Build history of the part. All positions in model axes, mm. Give positions to 0.01 mm unless a question says otherwise; leave off trailing zeros. Loops run counter-clockwise (first coordinate to the right, second up) from the corner with the lowest first, then second, coordinate; pieces in that order, holes last. Notation, with made-up numbers: M 38.5,-34 L 73.5,-34 A38 ccw 73.5,4 Z; hole C -34,-22 d1. An arc over 180 degrees is marked long. Answer as a JSON object with one key per item and string values. Group by question number.
1. Drop flat-ended pins along their axis: pin 1 Ø1.5 at (x, y) = (85, 3.5) entering from -Z; pin 2 Ø1.5 at (x, y) = (11.5, 3.5) entering from -Z; pin 3 Ø1.5 at (y, z) = (1, 7) entering from -X. Give the stop position or say it passes through.
2. Slice it at A-A (y = 3.1). Give the number of separate pieces and of enclosed holes in the cut face, then the cut area to 3 significant figures.
3. Drill centre lines: line 1 along X through (y, z) = (2.25, 0); line 2 along X through (y, z) = (0.9, 7); line 3 along X through (y, z) = (3.75, -6). Where is each one in solid material? Low to high. Write a range as [from, to].
4. Slice it at B-B (x = -36.5). List the corners of the cut face in (y, z), then the cut area to 3 significant figures.
from build123d import *

# Parameters (mm, degrees)
BOSS_EXTRUDE1_DEPTH = 5
SKETCH2_R           = 4
SKETCH2_R_2         = 1.5
CUT_EXTRUDE1_DEPTH  = 5
SKETCH3_R           = 1.5
CUT_EXTRUDE2_DEPTH  = 5
FILLET3_R           = 10
FILLET4_R           = 10


with BuildPart() as part:
    # Sketch1 → Boss-Extrude1 (new body)
    with BuildSketch(Plane(origin=(0, 0, 0), x_dir=(1, 0, 0), z_dir=(0, 1, 0))):
        Polygon((-85.638593384, 10), (-100, 10), (-100, -10), (-85.638593384, -10), (70, -10), (70, -15), (100, -15), (100, -10), (100, 10), (100, 15), (70, 15), (70, 10), align=None)
        with BuildLine():
            Line((-100, -10), (-100, 10))
            Line((-100, 10), (-85.638593384, 10))
            ThreePointArc((-85.638593384, 10), (-117.5, 0), (-85.638593384, -10))
            Line((-85.638593384, -10), (-100, -10))
        make_face()
    extrude(amount=BOSS_EXTRUDE1_DEPTH)

    # Sketch2 → Cut-Extrude1 (cut)
    with BuildSketch(Plane(origin=(0, 5, 0), x_dir=(1, 0, 0), z_dir=(0, 1, 0))):
        with Locations(Location((-99.485581351, 0, 0), (0, 0, 270))):
            Circle(SKETCH2_R)
        with Locations(Location((-99.485581351, 8, 0), (0, 0, 270))):
            Circle(SKETCH2_R_2)
        with Locations(Location((-99.485581351, -8, 0), (0, 0, 270))):
            Circle(SKETCH2_R_2)
        with Locations(Location((-108.985581351, 0, 0), (0, 0, 270))):
            Circle(SKETCH2_R_2)
        with Locations(Location((-89.985581351, 0, 0), (0, 0, 270))):
            Circle(SKETCH2_R_2)
    extrude(amount=-CUT_EXTRUDE1_DEPTH, mode=Mode.SUBTRACT)

    # Sketch3 → Cut-Extrude2 (cut)
    with BuildSketch(Plane(origin=(0, 5, 0), x_dir=(1, 0, 0), z_dir=(0, 1, 0))):
        with Locations(Location((77.928932188, 7.071067812, 0), (0, 0, 270))):
            Circle(SKETCH3_R)
        with Locations(Location((92.071067812, 7.071067812, 0), (0, 0, 270))):
            Circle(SKETCH3_R)
        with Locations(Location((92.071067812, -7.071067812, 0), (0, 0, 270))):
            Circle(SKETCH3_R)
        with Locations(Location((77.928932188, -7.071067812, 0), (0, 0, 270))):
            Circle(SKETCH3_R)
    extrude(amount=-CUT_EXTRUDE2_DEPTH, mode=Mode.SUBTRACT)

    # Fillet3
    # the kernel refuses this fillet: 10 mm, written as the material it takes off along each edge
    with BuildSketch(Plane(origin=(70, -21.650635095, 15), x_dir=(0, 0, -1), z_dir=(0, 1, 0))) as fillet3_piece_1:
        with BuildLine():
            CenterArc((10, -8.660254038), FILLET3_R, 120, 60)
            Line((0, -8.660254038), (-0.2, -8.660254038))
            Line((-0.2, -8.660254038), (-0.2, 0))
            Line((-0.2, 0), (0, 0.2))
            ThreePointArc((0, 0.2), (2.5, 0.2), (4.9, 0.173205081))
            Line((4.9, 0.173205081), (5, 0))
        make_face()
    extrude(amount=48.301270189, mode=Mode.SUBTRACT)
    with BuildSketch(Plane(origin=(100, -25, 15), x_dir=(0, 0, -1), z_dir=(0, 1, 0)), Plane(origin=(100, -25, -15), x_dir=(-1, 0, 0), z_dir=(0, 1, 0))) as fillet3_piece_2:
        with BuildLine():
            CenterArc((FILLET3_R, FILLET3_R), FILLET3_R, 180, 90)
            Line((0, FILLET3_R), (-FILLET3_R * 0.02, FILLET3_R))
            Line((-FILLET3_R * 0.02, FILLET3_R), (-FILLET3_R * 0.02, -FILLET3_R * 0.02))
            Line((-FILLET3_R * 0.02, -FILLET3_R * 0.02), (FILLET3_R, -FILLET3_R * 0.02))
            Line((FILLET3_R, -FILLET3_R * 0.02), (FILLET3_R, 0))
        make_face()
    extrude(amount=55, mode=Mode.SUBTRACT)
    with BuildSketch(Plane(origin=(70, -21.650635095, -15), x_dir=(0, 0, 1), z_dir=(0, 1, 0))) as fillet3_piece_3:
        with BuildLine():
            CenterArc((10, 8.660254038), FILLET3_R, 180, 60)
            Line((0, 8.660254038), (-0.2, 8.660254038))
            Line((-0.2, 8.660254038), (-0.2, 0))
            Line((-0.2, 0), (0, -0.2))
            ThreePointArc((0, -0.2), (2.5, -0.2), (4.9, -0.173205081))
            Line((4.9, -0.173205081), (5, 0))
        make_face()
    extrude(amount=48.301270189, mode=Mode.SUBTRACT)

    # Fillet4
    fillet4_edges = [part.edges().sort_by_distance(p)[0] for p in [
        (-85.638593384, 2.5, -10),
        (-85.638593384, 2.5, 10),
    ]]
    fillet(fillet4_edges, radius=FILLET4_R)


solid = part.part
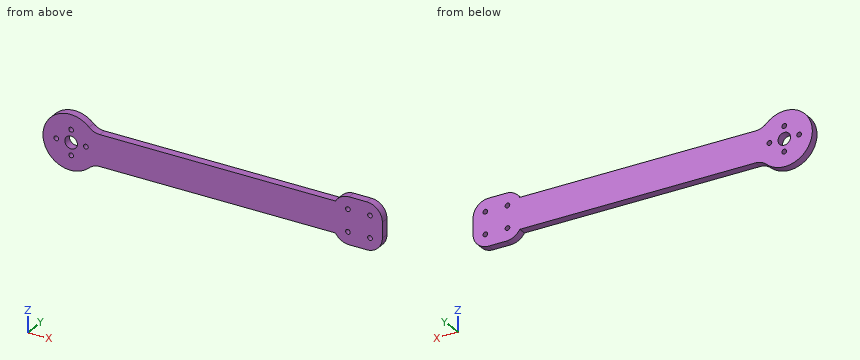
Established:
{
 "1": {"pin 1": "stops at z = -15", "pin 2": "stops at z = -10", "pin 3": "stops at x = -116.35"},
 "2": {"separate pieces": "1", "enclosed holes": "9", "area": "4,760 mm^2"},
 "3": {"line 1": "x = [-117.5, -110.49], [-107.49, -103.49], [-95.49, -91.49], [-88.49, 100]", "line 2": "x = [-116.04, -100.6], [-98.37, 76.43], [79.43, 90.57], [93.57, 99.8]", "line 3": "x = [-116.44, 76.88], [78.98, 91.02], [93.12, 99.95]"},
 "4": {"outline": "M 0,-10 L 5,-10 L 5,10 L 0,10 Z", "area": "100 mm^2"}
}
